Source: CAD feature listing. Evaluate the final solid. Frame: model axes, mm. Face numbers are marked on the shaded views. A direction names the side the tool comes from. Give positions to 0.01 mm unless a question says otherwise; leave off trailing zeros. Write each loop counter-clockwise with the first axis right and the second up, starting at its lowest first coordinate (ties: lowest second). Pieces come first, ordered by that corner, then holes. Notation, with made-up numbers: M 59.5,7 L 72.5,7 A14 cw 72.5,34 Z; hole C 81,32.25 d7. An arc over 180 degrees is marked long. Use CSV: the item, a comma, the result in double quotes. Start each with the question number.
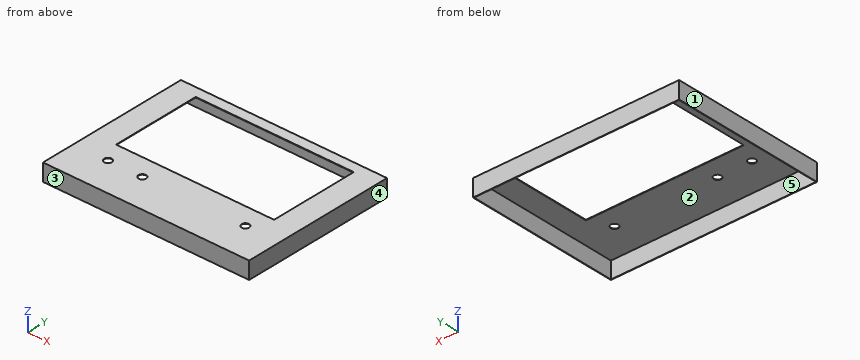
from build123d import *

# Parameters (mm, degrees)
SKETCH1_W           = 600
SKETCH1_H           = 450
BOSS_EXTRUDE1_DEPTH = 50
SHELL1_T            = -1.5
CUT_EXTRUDE1_REACH  = 52
SKETCH3_W           = 460
SKETCH3_H           = 260
CUT_EXTRUDE2_REACH  = 52
SKETCH4_R           = 11


with BuildPart() as part:
    # Sketch1 → Boss-Extrude1 (new body)
    with BuildSketch(Plane.XY):
        Rectangle(SKETCH1_W, SKETCH1_H)
    extrude(amount=BOSS_EXTRUDE1_DEPTH)

    # Shell1
    shell1_openings = [part.faces().sort_by_distance(p)[0] for p in [
        (0, 0, 0),
    ]]
    offset(amount=SHELL1_T, openings=shell1_openings, kind=Kind.INTERSECTION)

    # Sketch3 → Cut-Extrude1 (cut, up to next)
    with BuildSketch(Plane.XY.offset(50), mode=Mode.PRIVATE) as cut_extrude1_sk1:
        with Locations((0, 65)):
            Rectangle(SKETCH3_W, SKETCH3_H)
    cut_extrude1_tool1 = extrude(cut_extrude1_sk1.sketch, amount=-CUT_EXTRUDE1_REACH, mode=Mode.PRIVATE) & part.part
    add(cut_extrude1_tool1.solids().sort_by_distance((0, 65, 50))[0], mode=Mode.SUBTRACT)

    # Sketch4 → Cut-Extrude2 (cut, up to next)
    with BuildSketch(Plane.XY.offset(50), mode=Mode.PRIVATE) as cut_extrude2_sk1:
        with Locations((-200, -125)):
            Circle(SKETCH4_R)
    cut_extrude2_tool1 = extrude(cut_extrude2_sk1.sketch, amount=-CUT_EXTRUDE2_REACH, mode=Mode.PRIVATE) & part.part
    add(cut_extrude2_tool1.solids().sort_by_distance((-200, -125, 50))[0], mode=Mode.SUBTRACT)
    # Sketch4 → Cut-Extrude2 (cut, up to next)
    with BuildSketch(Plane.XY.offset(50), mode=Mode.PRIVATE) as cut_extrude2_sk2:
        with Locations((200, -125)):
            Circle(SKETCH4_R)
    cut_extrude2_tool2 = extrude(cut_extrude2_sk2.sketch, amount=-CUT_EXTRUDE2_REACH, mode=Mode.PRIVATE) & part.part
    add(cut_extrude2_tool2.solids().sort_by_distance((200, -125, 50))[0], mode=Mode.SUBTRACT)
    # Sketch4 → Cut-Extrude2 (cut, up to next)
    with BuildSketch(Plane.XY.offset(50), mode=Mode.PRIVATE) as cut_extrude2_sk3:
        with Locations((-100, -125)):
            Circle(SKETCH4_R)
    cut_extrude2_tool3 = extrude(cut_extrude2_sk3.sketch, amount=-CUT_EXTRUDE2_REACH, mode=Mode.PRIVATE) & part.part
    add(cut_extrude2_tool3.solids().sort_by_distance((-100, -125, 50))[0], mode=Mode.SUBTRACT)


solid = part.part
1. Access query for the marked faces 4 and 5. Directions: +Z, -Z, +X, -X, +Y, -Y. A direction counts if a zero-diameter tool reaches every point of the face in a straight line with its end or side. Return the directions, or none.
2. Section C-C on z = 33. Return loops of the section in (x, y), then the cut area to 3 significant figures.
3. Section D-D on y = -185. Return loops of the section in (x, z), then the cut area to 3 significant figures.
4. First-contact query: pin 1 (17.5 mm diameter, centred on x = 200, y = -125, fed in from +Z). Flat tip, straight axial feed; report the tip coordinate or a pass-through.
5. Pull-direction query (X, two-part tool) for the marked faces 1, 2 and 3; classes: released by +X, released by -X, zero draft, split by the parting line, or undercut.
6. Line query: probe 1 along Y at (x, z) = (200, 49); probe 2 along X at (y, z) = (177, 19.5); probe 3 along Y at (x, z) = (-100, 48). Output: solid intervals per line, ascending.
7. Section B-B on x = -100. Return loops of the section in (y, z).
8. Section A-A on y = -125. Return loops of the section in (x, z), then the cut area to 4 significant figures.
Resolved:
1,face 4,"+Z, -Z, +X, +Y, -Y"
1,face 5,"-Z"
2,outline,"M -300,-225 L 300,-225 L 300,225 L -300,225 Z; hole M -298.5,-223.5 L 298.5,-223.5 L 298.5,223.5 L -298.5,223.5 Z"
2,area,"3,140 mm2"
3,outline,"M -300,0 L -298.5,0 L -298.5,48.5 L 298.5,48.5 L 298.5,0 L 300,0 L 300,50 L -300,50 Z"
3,area,"1,050 mm2"
4,pin 1,"passes through"
5,face 1,"released by -X"
5,face 2,"undercut"
5,face 3,"zero draft"
6,probe 1,"y = -225 to -136, -114 to -65, 195 to 225"
6,probe 2,"x = -300 to -298.5, 298.5 to 300"
6,probe 3,"y = -225 to -223.5, 223.5 to 225"
7,outline,"M -225,0 L -223.5,0 L -223.5,48.5 L -136,48.5 L -136,50 L -225,50 Z; M -114,48.5 L -65,48.5 L -65,50 L -114,50 Z; M 195,48.5 L 223.5,48.5 L 223.5,0 L 225,0 L 225,50 L 195,50 Z"
8,outline,"M -300,0 L -298.5,0 L -298.5,48.5 L -211,48.5 L -211,50 L -300,50 Z; M -189,48.5 L -111,48.5 L -111,50 L -189,50 Z; M -89,48.5 L 189,48.5 L 189,50 L -89,50 Z; M 211,48.5 L 298.5,48.5 L 298.5,0 L 300,0 L 300,50 L 211,50 Z"
8,area,"946.5 mm2"
